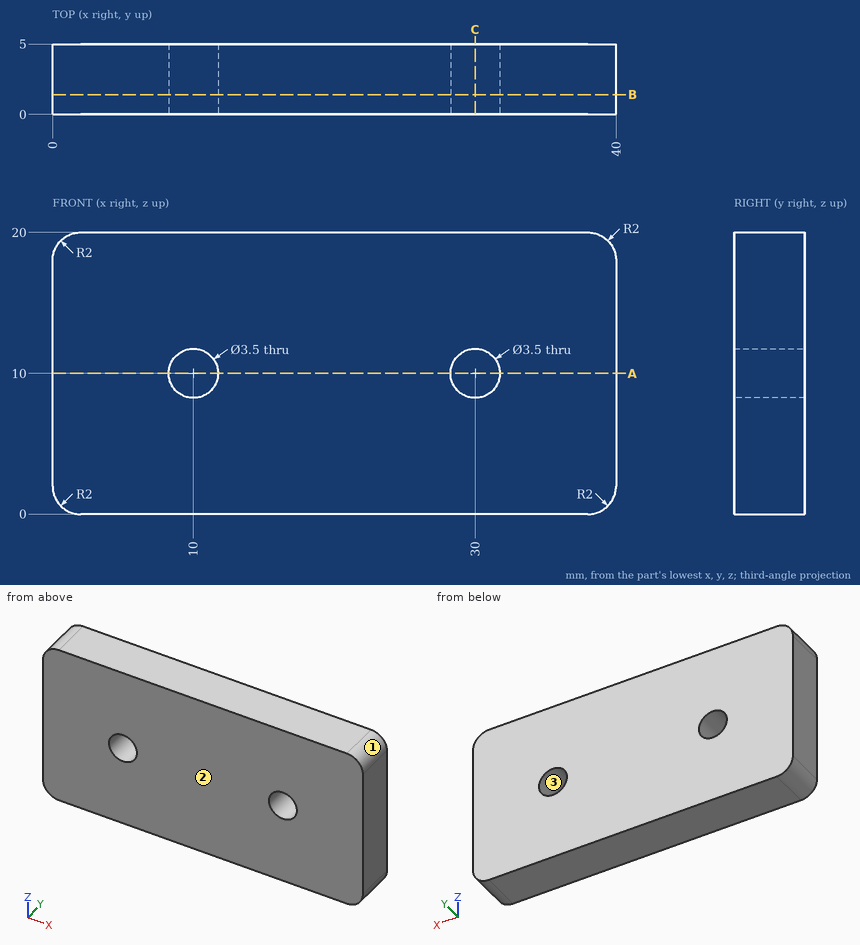
Study the drawing (mm; zero at the part's minimum x, y, z) and answer. Round coordinates to 2 decimals unless told otherwise and drop trailing zeros. Loops run counter-clockwise (first coordinate to the right, second up) from the corner with the lowest first, then second, coordinate; pieces in that order, holes last.
Q1. Section C-C, the plane x = 30 is taken. Determine the outline of the cut face in (y, z), then the cut area to 3 significant figures.
Q2. Section B-B, the plane y = 1.4 is taken. Determine the outline of the cut face in (x, z), then the cut area to 3 significant figures.
Q3. Find the intervals of material crossed by line 1 (X direction, y = 1.5, z = 10); line 2 (X direction, y = 1.4, z = 11); line 3 (Z direction, x = 29, y = 3.05), in increasing order.
Q4. Section A-A, the plane z = 10 is taken. Determine the outline of the cut face in (x, y), then the cut area to 3 significant figures.
Q5. For a pull along Z with two mould halves and no side action, classify the marked faces 1, 2 and 3 as released by +Z, released by -Z, zero draft, split by the parting line, or undercut.
Q6. Given pin 1 Ø3 at (x, z) = (10, 10) entering from -Y, flat-ended and moving along its own axis, determine where the tip first touches the part or whether it passes through.
Completed:
1. outline: (0, 0) - (5, 0) - (5, 8.25) - (0, 8.25) - close; (0, 11.75) - (5, 11.75) - (5, 20) - (0, 20) - close
1. area: 82.5 mm2
2. outline: (0, 2) arc R2 ccw to (2, 0) - (38, 0) arc R2 ccw to (40, 2) - (40, 18) arc R2 ccw to (38, 20) - (2, 20) arc R2 ccw to (0, 18) - close; hole circle Ø3.5 at (10, 10); hole circle Ø3.5 at (30, 10)
2. area: 777 mm2
3. line 1: x = 0 to 8.25, 11.75 to 28.25, 31.75 to 40
3. line 2: x = 0 to 8.56, 11.44 to 28.56, 31.44 to 40
3. line 3: z = 0 to 8.56, 11.44 to 20
4. outline: (0, 0) - (8.25, 0) - (8.25, 5) - (0, 5) - close; (11.75, 0) - (28.25, 0) - (28.25, 5) - (11.75, 5) - close; (31.75, 0) - (40, 0) - (40, 5) - (31.75, 5) - close
4. area: 165 mm2
5. face 1: released by +Z
5. face 2: zero draft
5. face 3: undercut
6. pin 1: passes through
